The listing builds one solid part. Answer for the finished solid, in the listing's coordinates (mm). A direction names the side the tool comes from. Give positions to 0.01 mm unless a question says otherwise; leave off trailing zeros. Order: outer loops, then holes, each group sorted by start corner. A loop starts at its lowest first (then second) coordinate and runs counter-clockwise, first axis right, second up. Notation, with made-up numbers: (65.25, 79) - (84.25, 79) arc R16 ccw to (84.25, 90) - close; hole circle Ø8 at (-24, -8.5). An arc over 180 degrees is marked (long way). Use CSV: the item, a comma, the result in double quotes.
```python
from build123d import *

# Parameters (mm, degrees)
CIRPATTERN1_COUNT = 4


with BuildPart() as part:
    # Sketch1 → Revolve1 (revolve)
    with BuildSketch(Plane.XY, mode=Mode.PRIVATE) as revolve1_sk:
        Polygon((0, 21), (11, 21), (11, 27.5), (37, 27.5), (37, 44), (5, 45), (5, 28), (0, 28), align=None)
    revolve(revolve1_sk.sketch.rotate(Axis((0, 0, 0), (1, 0, 0)), 90), axis=Axis((0, 0, 0), (1, 0, 0)))

    # Sketch4 → M8 Tapped Hole1 (revolve, cut)
    with BuildSketch(Plane(origin=(37, 35, 0), x_dir=(0, 0, -1), z_dir=(0, 1, 0))):
        Polygon((0, 0), (0, 24.292926105), (3.4, 22.25), (3.4, 0.625), (4.025, 0), align=None)
    m8_tapped_hole1 = revolve(axis=Axis((43.35, 35, 0), (-1, 0, 0)), mode=Mode.SUBTRACT)

    # CirPattern1: M8 Tapped Hole1 ×4 about axis
    cirpattern1_axis = Axis((0, 0, 0), (1, 0, 0))
    for i in range(1, CIRPATTERN1_COUNT):
        add(m8_tapped_hole1.rotate(cirpattern1_axis, i * 360 / CIRPATTERN1_COUNT), mode=Mode.SUBTRACT)


solid = part.part
```
Item 1: Find the intervals of material crossed by line 1 along Y through (x, z) = (24, 0); line 2 along Y through (x, z) = (28, 0); line 3 along Y through (x, z) = (4.25, 0), in increasing order.
Taken from the geometry:
line 1,"-44.41 to -38.4, -31.6 to -27.5, 27.5 to 31.6, 38.4 to 44.41"
line 2,"-44.28 to -38.4, -31.6 to -27.5, 27.5 to 31.6, 38.4 to 44.28"
line 3,"-28 to -21, 21 to 28"
Item 2: Each of these flat-tipped pins is pushed along its axis until it touches: pin 1 (8 mm diameter, centred on y = 0, z = -35, fed in from -X); pin 2 (1.5 mm diameter, centred on x = 6, z = -31, fed in from +Y); pin 3 (4 mm diameter, centred on y = -35, z = 0, fed in from +X). Where does it stop, or does it pass through?
Taken from the geometry:
pin 1,"x = 5"
pin 2,"y = 33.27"
pin 3,"x = 13.91"
Item 3: The part is cut by section A-A (x = 21). Give the vertices of the cut face in (y, z), and give its area (3 significant figures).
Taken from the geometry:
outline,"circle Ø89 at (0, 0); hole circle Ø6.8 at (-35, 0); hole circle Ø55 at (0, 0); hole circle Ø6.8 at (0, -35); hole circle Ø6.8 at (0, 35); hole circle Ø6.8 at (35, 0)"
area,"3,700 mm^2"
Item 4: The mould has two halves that part along Z. Classify faces 1 (the face through (2.46, 24.84, 12.92)), 2 (the face through (25.71, 31.63, 0.44)), 3 (the face through (0, -21, 4)): +Z half, -Z half, draft (parallel to the pull), parting line (faces both ways), or undercut.
Taken from the geometry:
face 1,"parting line"
face 2,"undercut"
face 3,"draft"
Item 5: Which of the six approach directions +Z, -Z, +X, -X, +Y, -Y give full straight-line access (tool end or side, diameter ignored) to faces 4 (the face through (25.714, -33.979, 3.243)), 5 (the face through (5.58, -6.31, 20.03)), 6 (the face through (5, 19, -21))?
Taken from the geometry:
face 4,"+X"
face 5,"+X, -X"
face 6,"-X"
